Autodesk Inventor part; units mm, degrees
ref_plane "YZ Plane" through (0, 0, 0) normal (1, 0, 0) x (0, 1, 0)
ref_plane "XZ Plane" through (0, 0, 0) normal (0, 1, 0) x (-1, 0, 0)
ref_plane "XY Plane" through (0, 0, 0) normal (0, 0, 1) x (1, 0, 0)
sketch "草圖1" plane through (0, 0, 0) normal (1, 0, 0) x (0, 1, 0)
  line L0 (0, 0) -> (45.4, 0)
  line L1 (45.4, 0) -> (45.4, -20)
  line L2 (45.4, -20) -> (40.4, -20)
  line L3 (40.4, -20) -> (0, -5)
  line L4 (0, -5) -> (0, 0)
  dimension "d0" = 45.4
  dimension "d1" = 20
  dimension "d2" = 5
  dimension "d3" = 5
extrude "擠出1" add sketch "草圖1" along normal mid plane 50
sketch "草圖2" plane through (25, 45.4, -20) normal (0, 0, -1) x (-1, 0, 0)
  line L0 (15, -12.7) -> (35, -12.7)
  line L1 (35, -12.7) -> (35, -32.7)
  line L2 (35, -32.7) -> (15, -32.7)
  line L3 (15, -32.7) -> (15, -12.7)
  line L4 (15, -12.7) -> (35, -32.7) construction
  line L5 (35, -12.7) -> (15, -32.7) construction
  line L6 (0, 0) -> (0, -45.4)
  point P0 (25, -45.4)
  point P1 (25, -22.7)
  point P2 (25, -22.7)
  point P3 (25, -22.7)
  point P4 (0, -22.7)
  dimension "d6" = 20
  dimension "d7" = 20
hole "孔1" at (10, 32.7, -20) at (10, 12.7, -20) at (-10, 12.7, -20) at (-10, 32.7, -20) direction (0, 0, 1) diameter 3.2 end through all counterbore diameter 5.7 counterbore depth 15
sketch "草圖3" plane through (-25, 45.4, 0) normal (0, 1, 0) x (1, 0, 0)
  line L0 (32.5, 15) -> (17.5, 15)
  line L1 (17.5, 15) -> (17.5, 5)
  line L2 (17.5, 5) -> (32.5, 5)
  line L3 (32.5, 5) -> (32.5, 15)
  line L4 (32.5, 15) -> (17.5, 5) construction
  line L5 (17.5, 15) -> (32.5, 5) construction
  line L6 (0, 0) -> (0, 20)
  line L7 (0, 20) -> (50, 20)
  point P0 (25, 0)
  point P1 (25, 10)
  point P2 (25, 10)
  point P3 (0, 10)
  point P4 (25, 10)
  point P5 (25, 20)
  dimension "d15" = 15
  dimension "d16" = 10
hole "孔2" at (7.5, 45.4, -5) at (-7.5, 45.4, -5) at (-7.5, 45.4, -15) at (7.5, 45.4, -15) direction (0, -1, 0) diameter 2.7 depth 10 counterbore diameter 4.1 counterbore depth 6
equation "\"d3\" = d2"
properties part number "線性滑塊轉接器"
Can you work these out from the model? Positions are in its coordinate system, mm. A direction names the side the tool comes from. Coordinates: 2 decimals unless noted, no trailing zeros. Order: outer loops, then holes, each group sorted by start corner. A loop starts at its lowest first (then second) coordinate and runs counter-clockwise, first axis right, second up. Notation, with made-up numbers: (-9, -32) - (10, -32) arc R25 cw to (10, -15) - close; hole circle Ø3 at (65, -32.5). An arc over 180 degrees is marked (long way). Answer as a JSON object with one key per item and string values. Group by question number.
Q1. We'd pull the mould along X, two halves only. Please class faces 4 (the face through (0, 0, -3)), 5 (the face through (6.161, 37.372, -5.176)), 6 (the face through (-25, 27, -8)), 7 (the face through (9, 39.4, -15)): +X half, -X half, draft (parallel to the pull), parting line (faces both ways), or undercut.
Q2. On a 3-axis mill with a long thin cutter (end or side, diameter ignored), from which of +Z, -Z, +X, -X, +Y, -Y can I reach the whole of each face in a straight line? I mean faces 1 (the face through (7.41, 42.36, -17.05)), 2 (the face through (-9.39, 14.18, -2.46)), 3 (the face through (12, 13, -5)). Say none if no direction works.
Q3. Imagine slicing it at B-B (z = -8). Please give me the cut outline in (x, y).
Q4. Imagine slicing it at C-C (z = -15). Please give me the cut outline in (x, y).
Q5. Imagine slicing it at D-D (x = 17.5). Please give me the cut outline in (y, z), and give its area (3 significant figures).
Q6. I need wall thicknesses on line 1 (X direction, y = 12.7, z = -7.8); line 2 (X direction, y = 43.1, z = -5); line 3 (Y direction, x = -10, z = -2.5). Which ranges of each line are inside material? Lowest first, please. Write a range as from..to.
Q7. Will these pins go through, and if not, where does the flat tip stop? P1, Ø10, axis at x = -13, y = 7.5, coming from the -Z side; P2, Ø1.2, axis at x = 7.5, z = -5, coming from the +Y side; P3, Ø3, axis at x = 7, y = 15.5, coming from the -Z side.
Q8. Imagine slicing it at A-A (y = 12.7). Please give me the cut outline in (x, z).
Determined:
{
 "1": {"face 4": "draft", "face 5": "undercut", "face 6": "-X half", "face 7": "undercut"},
 "2": {"face 1": "+Y", "face 2": "+Z, -Z", "face 3": "-Z"},
 "3": {"outline": "(-25, 8.08) - (25, 8.08) - (25, 45.4) - (-25, 45.4) - close; hole circle Ø5.7 at (-10, 12.7); hole circle Ø5.7 at (-10, 32.7); hole circle Ø5.7 at (10, 12.7); hole circle Ø5.7 at (10, 32.7)"},
 "4": {"outline": "(-25, 26.93) - (25, 26.93) - (25, 45.4) - (9.55, 45.4) - (9.55, 39.4) - (8.85, 39.4) - (8.85, 35.4) - (6.15, 35.4) - (6.15, 39.4) - (5.45, 39.4) - (5.45, 45.4) - (-5.45, 45.4) - (-5.45, 39.4) - (-6.15, 39.4) - (-6.15, 35.4) - (-8.85, 35.4) - (-8.85, 39.4) - (-9.55, 39.4) - (-9.55, 45.4) - (-25, 45.4) - close; hole circle Ø5.7 at (-10, 32.7); hole circle Ø5.7 at (10, 32.7)"},
 "5": {"outline": "(0, -5) - (40.4, -20) - (45.4, -20) - (45.4, 0) - (0, 0) - close", "area": "605 mm2"},
 "6": {"line 1": "x = -25..-12.85, -7.15..7.15, 12.85..25", "line 2": "x = -25..-9.55, -5.45..5.45, 9.55..25", "line 3": "y = 0..11.1, 14.3..31.1, 34.3..45.4"},
 "7": {"P1": "stops at z = -9.64", "P2": "stops at y = 35.4", "P3": "stops at z = -11.31"},
 "8": {"outline": "(-25, -9.72) - (-12.85, -9.72) - (-12.85, -5) - (-11.6, -5) - (-11.6, 0) - (-25, 0) - close; (-8.4, -5) - (-7.15, -5) - (-7.15, -9.72) - (7.15, -9.72) - (7.15, -5) - (8.4, -5) - (8.4, 0) - (-8.4, 0) - close; (11.6, -5) - (12.85, -5) - (12.85, -9.72) - (25, -9.72) - (25, 0) - (11.6, 0) - close"}
}
